For this review, take the finished solid that the model builds, in its own axes (mm). Face numbers are marked on the shaded views. Coordinates: 2 decimals unless noted, no trailing zeros. Loops run counter-clockwise (first coordinate to the right, second up) from the corner with the lowest first, then second, coordinate; pieces in that order, holes last.
1. Take a section at A-A, the plane z = 1.5. State the section outline as (x, y) points, then the cut area to 3 significant figures.
2. Clearance check with flat-ended pins moving along their axes: P1, Ø5, axis at x = 12.5, z = 5.34, coming from the +Y side; P2, Ø4, axis at y = -1.5, z = 8.5, coming from the +X side; P3, Ø4, axis at y = -2.5, z = 9.5, coming from the -X side; P4, Ø5.5, axis at x = -7, y = -8.5, coming from the +Z side. State where each tip first meets the part, or that it passes through.
3. To check wall thickness, follow probe 1 along X at (y, z) = (-6, -1.5); probe 2 along X at (y, z) = (-2, -3.5); probe 3 along Z at (x, y) = (13, -7.25). State the ranges of each line that lie inside material, in increasing order.
4. Take a section at B-B, the plane x = 15. State the section outline as (y, z) points.
5. Take a section at C-C, the plane y = -4.25. State the section outline as (x, z) points.
6. Take a section at D-D, the plane x = 0. State the section outline as (y, z) points.
7. Mouldability with a two-part tool opening along X and no side actions: class the marked faces 1, 2 and 3 as pulls with the +X half, pulls with the -X half, needs draft (parallel to the pull), parting line crosses it, or undercut.
```python
from build123d import *

# Parameters (mm, degrees)
F0_R     = 4.3187243864
F1_DEPTH = 11.43
F4_DEPTH = 25.4
F6_DEPTH = 25.4


# Not quite as in the source:
# - a pattern or mirror of a feature is missing from the dataset's text; its kind, count and spacing are read off the source's solid
# - the program builds the solid bodies; features that only make, move or delete a surface that nothing else refers to are left out


with BuildPart() as f1:
    # F0 (on Front) → F1 (new body)
    with BuildSketch(Plane.XZ):
        with BuildLine():
            ThreePointArc((-16.2297749531, -10.4286198462), (-16.1842309709, -10.4991606713), (-16.1383803934, -10.5695025995))
            ThreePointArc((-16.1383803934, -10.5695025995), (5.5149003864, -18.4864161116), (19.2914931232, 0))
            ThreePointArc((19.2914931232, 0), (-5.4343865811, 18.5102444449), (-16.2297749531, -10.4286198462))
        make_face()
        with Locations((-12.5015638769, 5.341576878)):
            Circle(F0_R, mode=Mode.SUBTRACT)
        with Locations((12.5015638769, 5.341576878)):
            Circle(F0_R, mode=Mode.SUBTRACT)
    extrude(amount=F1_DEPTH)

    # F2 (on Front) → F4 (cut)
    with BuildSketch(Plane.XZ):
        with BuildLine():
            Line((-15.6837776303, -10.0077530369), (14.2410276458, -10.0077530369))
            ThreePointArc((14.2410276458, -10.0077530369), (-0.7213749923, -3.7564431571), (-15.6837776303, -10.0077530369))
        make_face()
    extrude(amount=F4_DEPTH, mode=Mode.SUBTRACT)

    # F5 (on face) → F6 (cut)
    with BuildSketch(Plane.XZ.offset(11.43)):
        with BuildLine():
            Line((-11.7404377088, -3.5014220048), (-11.7787355557, 0))
            Line((-11.7787355557, 0), (-13.1083335727, -2.8944755904))
            ThreePointArc((-13.1083335727, -2.8944755904), (-12.7318294924, -3.8908455066), (-11.7404377088, -3.5014220048))
        make_face()
    f6 = extrude(amount=-F6_DEPTH, mode=Mode.SUBTRACT)

    # F6_copies: F6 across plane
    add(f6.mirror(Plane(origin=(0, 0, 0), x_dir=(0, 0, 1), z_dir=(1, 0, 0))), mode=Mode.SUBTRACT)


solid = f1.part
```
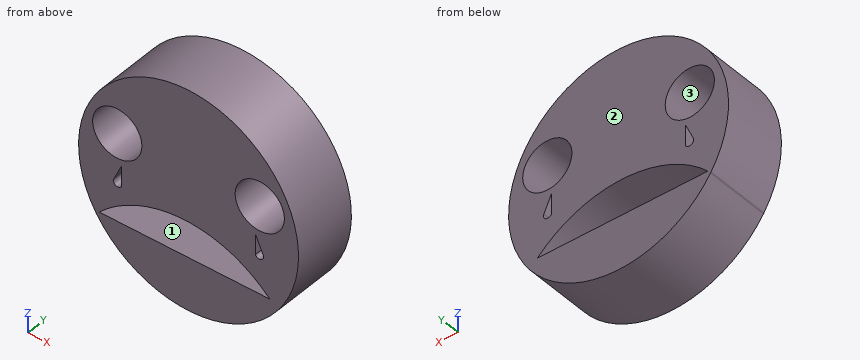
Results list:
1. outline: (-19.23, -11.43) - (-14.47, -11.43) - (-14.47, 0) - (-19.23, 0) - close; (-10.53, -11.43) - (10.53, -11.43) - (10.53, 0) - (-10.53, 0) - close; (14.47, -11.43) - (19.23, -11.43) - (19.23, 0) - (14.47, 0) - close
1. area: 349 mm2
2. P1: passes through
2. P2: stops at x = 18.16
2. P3: stops at x = -17.77
2. P4: stops at z = 18.82
3. probe 1: x = -19.23 to -12.47, -11.76 to 11.76, 12.47 to 19.23
3. probe 2: x = -18.97 to -13.12, -11.74 to 11.74, 13.12 to 18.97
3. probe 3: z = -14.25 to -10.01, -8.85 to -3.69, -2.66 to 1.05, 9.63 to 14.25
4. outline: (-11.43, -12.13) - (0, -12.13) - (0, 1.82) - (-11.43, 1.82) - close; (-11.43, 8.86) - (0, 8.86) - (0, 12.13) - (-11.43, 12.13) - close
5. outline: (-16.23, -10.43) arc R19.29 ccw to (-16.14, -10.57) arc R19.29 ccw (long way) to start; hole circle Ø8.64 at (-12.5, 5.34); hole (-15.68, -10.01) - (14.24, -10.01) arc R21.03 ccw to start; hole (-13.11, -2.89) arc R0.75 ccw (long way) to (-11.74, -3.5) - (-11.78, 0) - close; hole circle Ø8.64 at (12.5, 5.34); hole (11.74, -3.5) arc R0.75 ccw (long way) to (13.11, -2.89) - (11.78, 0) - close
6. outline: (-11.43, -19.29) - (0, -19.29) - (0, -10.01) - (-11.43, -10.01) - close; (-11.43, -3.77) - (0, -3.77) - (0, 19.29) - (-11.43, 19.29) - close
7. face 1: undercut
7. face 2: needs draft
7. face 3: undercut
